Check sheet for the modelled part. Datum: model origin and axes. Units: mm. A direction names the side the tool comes from. Give positions to 0.01 mm unless a question says otherwise; leave off trailing zeros. Write each loop counter-clockwise with the first axis right and the second up, starting at its lowest first coordinate (ties: lowest second). Pieces come first, ordered by that corner, then holes. Notation, with made-up numbers: M 15,68 L 24,68 A4 ccw 24,75 Z; hole C 76.5,71.25 d1. An arc over 180 degrees is marked long. Write each question's results on one line, items separated by ' | '. Start each with the question number.
Autodesk Inventor part; units mm, degrees
ref_plane "YZ Plane" through (0, 0, 0) normal (1, 0, 0) x (0, 1, 0)
ref_plane "XZ Plane" through (0, 0, 0) normal (0, 1, 0) x (-1, 0, 0)
ref_plane "XY Plane" through (0, 0, 0) normal (0, 0, 1) x (1, 0, 0)
sketch "Sketch1" plane through (0, 0, 0) normal (1, 0, 0) x (0, 1, 0)
  line L0 (128.3979, 81.9005) -> (-112.6021, 81.9005)
  line L1 (-112.6021, 81.9005) -> (-112.6021, -0.0995)
  line L2 (-112.6021, -0.0995) -> (128.3979, -0.0995)
  line L3 (128.3979, -0.0995) -> (128.3979, 81.9005)
  circle A0 centre (-45.6021, 40.9005) radius 19 construction
  line L4 (-112.6021, 73.9005) -> (-109.6021, 73.9005)
  line L5 (-109.6021, 73.9005) -> (-109.6021, 7.9005)
  line L6 (-109.6021, 7.9005) -> (-112.6021, 7.9005)
  line L7 (-112.6021, 7.9005) -> (-112.6021, 73.9005)
  circle A1 centre (111.4349, 69.7734) radius 2.5
  point P0 (0, 0)
  dimension "d0" = 241
  dimension "d1" = 82
  dimension "d2" = 38
  dimension "d3" = 41
  dimension "d4" = 174
  dimension "d5" = 66
  dimension "d6" = 3
  dimension "d7" = 8
  dimension "d24" = 5
extrude "Extrusion3" add sketch "Sketch1" along normal blind 5 contours L3 L2 L1 L6 L5 L4 L0 | A1
sketch "Sketch3" plane through (5, 0, 0) normal (1, 0, 0) x (0, 0, -1)
  circle A0 centre (-65.9005, 108.8979) radius 2.5
  line L0 (-81.9005, 128.3979) -> (-81.9005, -112.6021)
  line L1 (-81.9005, 128.3979) -> (-74.525, 128.3979) construction
  line L2 (-81.9005, 122.7969) -> (-81.9005, 128.3979) construction
  circle A1 centre (-15.9005, 108.8979) radius 2.5
  circle A2 centre (-65.9005, 58.8979) radius 2.5
  circle A3 centre (-15.9005, 58.8979) radius 2.5
  line L3 (0.0995, -112.6021) -> (0.0995, 128.3979)
  line L4 (0.0995, 128.3979) -> (-81.9005, 128.3979)
  point P0 (0, 0)
  dimension "d25" = 5
  dimension "d28" = 50
  dimension "d31" = 50
  dimension "d34" = 82
  dimension "d35" = 16
  dimension "d36" = 19.5
extrude "Extrusion4" cut sketch "Sketch3" against normal up to surface (5 mm away)
sketch "Sketch4" plane through (5, 0, 0) normal (1, 0, 0) x (0, 0, -1)
  circle A0 centre (-40.9005, -65.6021) radius 19
  line L0 (-73.9005, -109.6021) -> (-7.9005, -109.6021)
  point P0 (0, 0)
  point P1 (-40.9005, -109.6021)
  dimension "d39" = 38
  dimension "d40" = 44
extrude "Extrusion5" cut sketch "Sketch4" against normal up to surface (5 mm away)
pattern_linear "Rectangular Pattern1" count 2 spacing 50 along (0, 1, 0) of "Extrusion5"
equation "\"d3\" = 0.5 * d1"
equation "\"d7\" = -0.5 * d5 + 0.5 * d1"
equation "\"d35\" = -0.5 * d28 + 0.5 * d34"
properties part number "center_2Poke"
Q1. Section check B-B on z = 66. Record the boundary of the cut face in (x, y).
Q2. Depth check by flat-ended pin: pin 1 Ø4.5 at (y, z) = (108.9, 15.9) entering from +X; pin 2 Ø2.5 at (x, z) = (2.5, 51) entering from -Y. Enter the tip coordinate at first touch or a pass-through.
Q3. Section check D-D on z = 33.5. Record the boundary of the cut face in (x, y).
Q4. Section check A-A on y = -26.5. Record the boundary of the cut face in (x, z), plus the area to 3 significant figures.
Q5. Scan lines: L1, parallel to Y at x = 0.4, z = 24; L2, parallel to Y at x = 1.2, z = 17.5; L3, parallel to Y at x = 1.85, z = 68.5. Record each from-to range of solid material in increasing order.
Q6. Release check for a two-part mould opening along Z. For faces 1 (the face through (2.535, -59.895, 22.778)), 2 (the face through (2, 10, 81.9)), 3 (the face through (2.535, 56.457, 16.442)), 4 (the face through (5, 6, 41)) record: pulls with the +Z half, pulls with the -Z half, needs draft (parallel to the pull), parting line crosses it, or undercut.
Q7. Section check C-C on x = 1.7. Record the boundary of the cut face in (y, z).
Q8. Tool access check on faces 5 (the face through (2, -109.602, 41)), 6 (the face through (2, -112.602, 4)). Record the directions out of +Z, -Z, +X, -X, +Y, -Y that give a thin tool (end or side, any length) a straight path to the whole face; none if there is none.
Check result:
1) outline: M 0,-109.6 L 5,-109.6 L 5,56.4 L 0,56.4 Z; M 0,61.4 L 5,61.4 L 5,106.4 L 0,106.4 Z; M 0,111.4 L 5,111.4 L 5,128.4 L 0,128.4 Z
2) pin 1: through | pin 2: y = -109.6
3) outline: M 0,-109.6 L 5,-109.6 L 5,-83.1 L 0,-83.1 Z; M 0,-48.1 L 5,-48.1 L 5,-33.1 L 0,-33.1 Z; M 0,1.9 L 5,1.9 L 5,128.4 L 0,128.4 Z
4) outline: M 0,-0.1 L 5,-0.1 L 5,25.34 L 0,25.34 Z; M 0,56.46 L 5,56.46 L 5,81.9 L 0,81.9 Z | area: 254 mm^2
5) L1: -109.6 to -74.28, -56.92 to -24.28, -6.92 to 128.4 | L2: -109.6 to 56.98, 60.82 to 106.98, 110.82 to 128.4 | L3: -109.6 to 128.4
6) face 1: undercut | face 2: pulls with the +Z half | face 3: undercut | face 4: needs draft
7) outline: M -112.6,-0.1 L 128.4,-0.1 L 128.4,81.9 L -112.6,81.9 L -112.6,73.9 L -109.6,73.9 L -109.6,7.9 L -112.6,7.9 Z; hole C -65.6,40.9 d38; hole C -15.6,40.9 d38; hole C 58.9,15.9 d5; hole C 58.9,65.9 d5; hole C 108.9,15.9 d5; hole C 108.9,65.9 d5
8) face 5: +X, -X, -Y | face 6: +Z, -Z, +X, -X, -Y
